```python
from build123d import *


with BuildPart() as f1:
    # F0 (on Front) → F1 (revolve)
    with BuildSketch(Plane.XZ):
        with BuildLine():
            Line((-5, 0), (0, 0))
            Line((0, 0), (0, 7))
            ThreePointArc((0, 7), (-1.113366, 12.047892), (-4.246868, 16.159091))
            ThreePointArc((-4.246868, 16.159091), (-7.871386, 18.267411), (-12, 19))
            ThreePointArc((-12, 19), (-19.071068, 21.928932), (-22, 29))
            Line((-22, 29), (-22, 100))
            Line((-22, 100), (-27, 100))
            Line((-27, 100), (-27, 29))
            ThreePointArc((-27, 29), (-22.606602, 18.393398), (-12, 14))
            ThreePointArc((-12, 14), (-7.050253, 11.949747), (-5, 7))
            Line((-5, 7), (-5, 0))
        make_face()
    revolve(axis=Axis((17, 0, 30.384544), (0, 0, 1)))


solid = f1.part
```
The listing builds one solid part. Answer for the finished solid, in the listing's coordinates (mm). A direction names the side the tool comes from. Give positions to 0.01 mm unless a question says otherwise; leave off trailing zeros. Order: outer loops, then holes, each group sorted by start corner. A loop starts at its lowest first (then second) coordinate and runs counter-clockwise, first axis right, second up. Notation, with made-up numbers: (73.5, 26) -> (116.5, 26) arc R19 ccw to (116.5, 40) -> close; hole circle Ø3 at (33.5, 36). An arc over 180 degrees is marked (long way). Answer as a JSON object with one key per item and string values. Group by question number.
Item 1: A tool of negligible diameter and unlimited length cuts with its end or side. For faces 4 (the cylindrical face through (22.077, -38.668, 64.997)), 5 (the flat face through (5.7, 12.93, 0)), from which of +Z, -Z, +X, -X, +Y, -Y can it reach the whole face along a straight path? Write none if from no direction.
Item 2: Consider L1, parallel to Y at x = 17, z = 45; L2, parallel to X at y = 0, z = 2; L3, parallel to X at y = 0, z = 69. Determine where each line is inside the solid, lowest interval first. Write a range as from..to.
Item 3: The part is cut by section C-C on z = 85.5. Write down the section's boundary in (x, y).
Item 4: Flat-ended cylindrical pins translate along their axes: pin 1 (8 mm diameter, centred on x = -1.5, z = 47.5, fed in from +Y); pin 2 (10 mm diameter, centred on x = 10.5, y = -31.5, fed in from +Z); pin 3 (1 mm diameter, centred on x = -0.5, y = 18, fed in from -Z). Find the tip coordinate at first contact, or state that the pin passes through.
Item 5: The part is cut by section A-A on x = 17. Write down the section's boundary in (y, z), and give its area (3 significant figures).
Item 6: Determine the mould class of faces 1 (the flat face through (-9.3, 29.1, 100)), 2 (the cylindrical face through (21.769, 21.477, 3.451)), 3 (the cylindrical face through (29.53, -11.49, 3.55)) for opening direction X: pulls with the +X half, pulls with the -X half, needs draft (parallel to the pull), parting line crosses it, or undercut.
Item 7: The part is cut by section D-D on z = 25. Write down the section's boundary in (x, y).
Item 8: The part is cut by section B-B on y = 0. Write down the section's boundary in (x, z), and give its area (3 significant figures).
Result set:
{
 "1": {"face 4": "+Z", "face 5": "-Z, +X, -X, +Y, -Y"},
 "2": {"L1": "-44..-39, 39..44", "L2": "-5..0, 34..39", "L3": "-27..-22, 56..61"},
 "3": {"outline": "circle Ø88 at (17, 0); hole circle Ø78 at (17, 0)"},
 "4": {"pin 1": "y = 41.54", "pin 2": "z = 23.22", "pin 3": "z = 12.45"},
 "5": {"outline": "(-44, 29) arc R15 ccw to (-29, 14) arc R7 cw to (-22, 7) -> (-22, 0) -> (-17, 0) -> (-17, 7) arc R12 ccw to (-21.25, 16.16) arc R12 ccw to (-29, 19) arc R10 cw to (-39, 29) -> (-39, 100) -> (-44, 100) -> close; (17, 0) -> (22, 0) -> (22, 7) arc R7 cw to (29, 14) arc R15 ccw to (44, 29) -> (44, 100) -> (39, 100) -> (39, 29) arc R10 cw to (29, 19) arc R12 ccw to (21.25, 16.16) arc R12 ccw to (17, 7) -> close", "area": "1,130 mm²"},
 "6": {"face 1": "needs draft", "face 2": "parting line crosses it", "face 3": "undercut"},
 "7": {"outline": "circle Ø86.91 at (17, 0); hole circle Ø76.33 at (17, 0)"},
 "8": {"outline": "(-27, 29) arc R15 ccw to (-12, 14) arc R7 cw to (-5, 7) -> (-5, 0) -> (0, 0) -> (0, 7) arc R12 ccw to (-4.25, 16.16) arc R12 ccw to (-12, 19) arc R10 cw to (-22, 29) -> (-22, 100) -> (-27, 100) -> close; (34, 0) -> (39, 0) -> (39, 7) arc R7 cw to (46, 14) arc R15 ccw to (61, 29) -> (61, 100) -> (56, 100) -> (56, 29) arc R10 cw to (46, 19) arc R12 ccw to (38.25, 16.16) arc R12 ccw to (34, 7) -> close", "area": "1,130 mm²"}
}
